Can you work these out from the model? Positions are in its coordinate system, mm. Coordinates: 2 decimals unless noted, no trailing zeros. Order: outer loops, then holes, each group sorted by start corner. A loop starts at its lowest first (then second) coordinate and runs counter-clockwise, first axis right, second up. Notation, with made-up numbers: (9.5, 61.25) -> (14.5, 61.25) arc R17 ccw to (14.5, 92.25) -> close; hole circle Ø1 at (8, -21). An arc over 180 degrees is marked (long way). Answer as CSV lines item,"result".
Autodesk Inventor part; units mm, degrees
ref_plane "YZ Plane" through (0, 0, 0) normal (1, 0, 0) x (0, 1, 0)
ref_plane "XZ Plane" through (0, 0, 0) normal (0, 1, 0) x (-1, 0, 0)
ref_plane "XY Plane" through (0, 0, 0) normal (0, 0, 1) x (1, 0, 0)
sketch "Sketch1" plane through (0, 0, 0) normal (0, 1, 0) x (-1, 0, 0)
  line L0 (-20, 40) -> (20, 40)
  line L1 (20, 40) -> (20, -40)
  line L2 (20, -40) -> (-20, -40)
  line L3 (-20, -40) -> (-20, 40)
  line L4 (-20, 40) -> (20, -40) construction
  line L5 (20, 40) -> (-20, -40) construction
  line L6 (-18.75, 38.75) -> (18.75, 38.75)
  line L7 (18.75, 38.75) -> (18.75, -38.75)
  line L8 (18.75, -38.75) -> (-18.75, -38.75)
  line L9 (-18.75, -38.75) -> (-18.75, 38.75)
  line L10 (-18.75, 38.75) -> (18.75, -38.75) construction
  line L11 (18.75, 38.75) -> (-18.75, -38.75) construction
  point P0 (0, 0)
  dimension "d0" = 40
  dimension "d1" = 80
  dimension "d2" = 37.5
  dimension "d19" = 77.5
extrude "Extrusion1" add sketch "Sketch1" along normal blind 1824.7
fillet "Fillet1" radius 2.5 4 edges at (-18.75, 912.35, 38.75) (18.75, 912.35, -38.75) (18.75, 912.35, 38.75) (-18.75, 912.35, -38.75)
fillet "Fillet1" radius 3.75 4 edges at (20, 912.35, 40) (-20, 912.35, 40) (20, 912.35, -40) (-20, 912.35, -40)
sketch "Boceto3" plane through (-16.25, 0, 40) normal (0, 0, 1) x (1, 0, 0)
  circle A0 centre (16, 11.25) radius 4.5
  circle A1 centre (16, 68.75) radius 4.5
  circle A2 centre (16, 911.25) radius 4.5
  circle A3 centre (16, 968.75) radius 4.5
  circle A4 centre (16, 1268.75) radius 4.5
  circle A5 centre (16, 1211.25) radius 4.5
  circle A6 centre (16, 11.25) radius 5.5
  circle A7 centre (16, 68.75) radius 5.5
  circle A8 centre (16, 911.25) radius 5.5
  circle A9 centre (16, 968.75) radius 5.5
  circle A10 centre (16, 1268.75) radius 5.5
  circle A11 centre (16, 1211.25) radius 5.5
  point P0 (16.25, 0)
  dimension "d11" = 11
  dimension "d12" = 11
  dimension "d13" = 11
  dimension "d14" = 11
  dimension "d15" = 11
  dimension "d16" = 11
extrude "Extrusión3" cut sketch "Boceto3" against normal blind 10 contours A0 | A1 | A2 | A3 | A4 | A5 | A6 | A7 | A8 | A9 | A10 | A11
sketch "Sketch6" plane through (-20, 0, -36.25) normal (-1, 0, 0) x (0, 0, 1)
  point P0 (36.25, 0)
sketch "Sketch8" plane through (-20, 0, -36.25) normal (-1, 0, 0) x (0, 0, 1)
  circle A0 centre (24.3846, 1771.4414) radius 11.11
  point P0 (36.25, 0)
extrude "Extrusion7" cut sketch "Sketch8" against normal through all
properties part number "tubo1-40x40x1800" material "Acero, carbono"
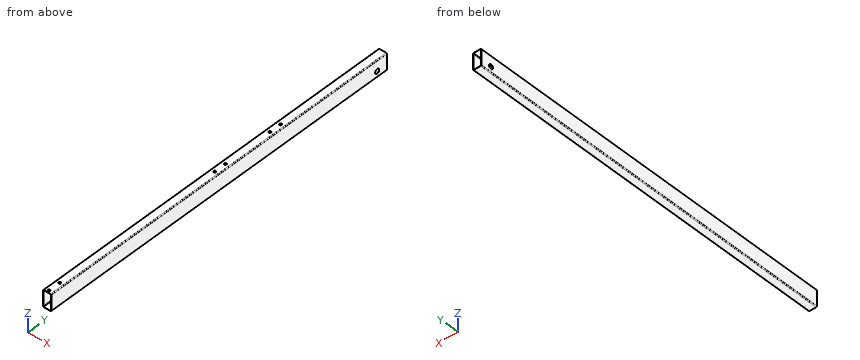
Q1. For P1, Ø9, axis at x = -0.25, y = 11.25, coming from the +Z side, with a flat end and sliding along its axis, tell me the tip position at first contact or that it passes through.
Solution:
P1,"z = -38.75"
Q2. Imagine slicing it at B-B (y = 478.5). List the corners of the cut face in (x, z) for me, and give its area (3 significant figures).
Solution:
outline,"(-20, -36.25) arc R3.75 ccw to (-16.25, -40) -> (16.25, -40) arc R3.75 ccw to (20, -36.25) -> (20, 36.25) arc R3.75 ccw to (16.25, 40) -> (-16.25, 40) arc R3.75 ccw to (-20, 36.25) -> close; hole (-18.75, -36.25) arc R2.5 ccw to (-16.25, -38.75) -> (16.25, -38.75) arc R2.5 ccw to (18.75, -36.25) -> (18.75, 36.25) arc R2.5 ccw to (16.25, 38.75) -> (-16.25, 38.75) arc R2.5 ccw to (-18.75, 36.25) -> close"
area,"287 mm2"
Q3. If I drill on line 1 (Z direction, x = -17, y = 970); line 2 (Z direction, x = 12, y = 1688); line 3 (X direction, y = 746, z = 8.5), over which ranges is the centre line in solid material (lowest first)?
Solution:
line 1,"-39.92 to -38.63, 38.63 to 39.92"
line 2,"-40 to -38.75, 38.75 to 40"
line 3,"-20 to -18.75, 18.75 to 20"
Q4. Imagine slicing it at A-A (z = 22.5). List the corners of the cut face in (x, y) for me.
Solution:
outline,"(-20, 0) -> (-18.75, 0) -> (-18.75, 1824.7) -> (-20, 1824.7) -> close; (18.75, 0) -> (20, 0) -> (20, 1824.7) -> (18.75, 1824.7) -> close"
